```python
from build123d import *

# Parameters (mm, degrees)
SKETCH1_R               = 22.5
SKETCH1_R_2             = 20
BOSS_EXTRUDE1_DEPTH     = 30
BOSS_EXTRUDE2_DEPTH     = 4
CHAMFER1_SIZE           = 2
CHAMFER1_SIZE_2         = 1.79025908
CUT_EXTRUDE1_DEPTH      = 39.684622268
CUT_EXTRUDE1_DEPTH_BACK = 39.684622268
BOSS_EXTRUDE3_START     = -1.5
BOSS_EXTRUDE3_DEPTH     = 1.5
SKETCH6_R               = 13.5
SKETCH6_R_2             = 11.05
BOSS_EXTRUDE4_DEPTH     = 8
CHAMFER2_SIZE           = 1
CHAMFER3_SIZE           = 1
CHAMFER4_SIZE           = 2.5


with BuildPart() as part:
    # Sketch1 → Boss-Extrude1 (new body)
    with BuildSketch(Plane(origin=(0, 0, 0), x_dir=(1, 0, 0), z_dir=(0, 1, 0))):
        with Locations(Location((0, 0, 0), (0, 0, 270))):
            Circle(SKETCH1_R)
        with Locations(Location((0, 0, 0), (0, 0, 270))):
            Circle(SKETCH1_R_2, mode=Mode.SUBTRACT)
    extrude(amount=BOSS_EXTRUDE1_DEPTH)

    # Sketch2 → Boss-Extrude2 (add, symmetric)
    with BuildSketch(Plane(origin=(0, 18, 0), x_dir=(1, 0, 0), z_dir=(0, 1, 0))):
        with BuildLine():
            Line((-12.086630926, 15.934658856), (-4.330127019, 2.5))
            Line((-4.330127019, 2.5), (-19.843134833, 2.5))
            ThreePointArc((-19.843134833, 2.5), (-20, 0), (-19.843134833, -2.5))
            Line((-19.843134833, -2.5), (-4.330127019, -2.5))
            Line((-4.330127019, -2.5), (-12.086630926, -15.934658856))
            ThreePointArc((-12.086630926, -15.934658856), (-10, -17.320508076), (-7.756503907, -18.434658856))
            Line((-7.756503907, -18.434658856), (0, -5))
            Line((0, -5), (7.756503907, -18.434658856))
            ThreePointArc((7.756503907, -18.434658856), (10, -17.320508076), (12.086630926, -15.934658856))
            Line((12.086630926, -15.934658856), (4.330127019, -2.5))
            Line((4.330127019, -2.5), (19.843134833, -2.5))
            ThreePointArc((19.843134833, -2.5), (19.960745185, -1.252458251), (20, 0))
            ThreePointArc((20, 0), (19.960745185, 1.252458251), (19.843134833, 2.5))
            Line((19.843134833, 2.5), (4.330127019, 2.5))
            Line((4.330127019, 2.5), (12.086630926, 15.934658856))
            ThreePointArc((12.086630926, 15.934658856), (10, 17.320508076), (7.756503907, 18.434658856))
            Line((7.756503907, 18.434658856), (0, 5))
            Line((0, 5), (-7.756503907, 18.434658856))
            ThreePointArc((-7.756503907, 18.434658856), (-10, 17.320508076), (-12.086630926, 15.934658856))
        make_face()
    extrude(amount=BOSS_EXTRUDE2_DEPTH, both=True)

    # Chamfer1
    # the kernel refuses this chamfer: 2, 1.79025908 mm, written as the material it adds along each edge
    with BuildSketch(Plane(origin=(7.756503907, 22, 18.434658856), x_dir=(-0.9376749432180777, 0, 0.34751359809505994), z_dir=(0, -1, 0)), Plane(origin=(19.843134833, 22, 2.5), x_dir=(-0.16788186749818226, 0, 0.9858071203665161), z_dir=(0, -1, 0)), Plane(origin=(12.086630926, 22, -15.934658856), x_dir=(0.7697930757198956, 0, 0.6382935222714571), z_dir=(0, -1, 0)), Plane(origin=(-7.756503907, 22, -18.434658856), x_dir=(0.9376749432180783, 0, -0.34751359809505833), z_dir=(0, -1, 0)), Plane(origin=(-19.843134833, 22, -2.5), x_dir=(0.1678818674981782, 0, -0.9858071203665167), z_dir=(0, -1, 0)), Plane(origin=(-12.086630926, 22, 15.934658856), x_dir=(-0.7697930757198955, 0, -0.6382935222714572), z_dir=(0, -1, 0))) as chamfer1_piece_1:
        with BuildLine():
            Line((1.733569464, 0), (CHAMFER1_SIZE * 0.167881867498, CHAMFER1_SIZE * 0.985807120367))
            Line((CHAMFER1_SIZE * 0.167881867498, CHAMFER1_SIZE * 0.985807120367), (0, 0))
            ThreePointArc((0, 0), (0.889903139, -0.018778361), (1.733569464, 0))
        make_face()
    extrude(amount=8)
    with BuildSketch(Plane(origin=(12.086630926, 14, 15.934658856), x_dir=(0.7669529363679002, 0, -0.6417033531131466), z_dir=(0, 1, 0)), Plane(origin=(19.843134833, 14, -2.5), x_dir=(-0.17225493730569186, 0, -0.9850524029582447), z_dir=(0, 1, 0)), Plane(origin=(7.756503907, 14, -18.434658856), x_dir=(-0.9392078736735914, 0, -0.3433490498450975), z_dir=(0, 1, 0)), Plane(origin=(-12.086630926, 14, -15.934658856), x_dir=(-0.766952936367899, 0, 0.641703353113148), z_dir=(0, 1, 0)), Plane(origin=(-19.843134833, 14, 2.5), x_dir=(0.17225493730568892, 0, 0.9850524029582453), z_dir=(0, 1, 0)), Plane(origin=(-7.756503907, 14, 18.434658856), x_dir=(0.9392078736735913, 0, 0.3433490498450977), z_dir=(0, 1, 0))) as chamfer1_piece_2:
        with BuildLine():
            Line((1.910893878, 0), (CHAMFER1_SIZE_2 * 0.172254937261, CHAMFER1_SIZE_2 * 0.985052402702))
            Line((CHAMFER1_SIZE_2 * 0.172254937261, CHAMFER1_SIZE_2 * 0.985052402702), (0, 0))
            ThreePointArc((0, 0), (0.982338586, -0.022816928), (1.910893878, 0))
        make_face()
    extrude(amount=8)

    # Sketch4 → Cut-Extrude1 (cut, two sides: drawn at the far end of the back side and taken through both)
    with BuildSketch(Plane(origin=(0, 22, 0), x_dir=(1, 0, 0), z_dir=(0, 1, 0)).offset(-CUT_EXTRUDE1_DEPTH_BACK)):
        with BuildLine():
            Line((-1.09656677, 1.165135752), (-1.097544149, 0.833904576))
            Line((-1.097544149, 0.833904576), (-1.102446274, -0.827412964))
            Line((-1.102446274, -0.827412964), (-1.103423653, -1.15864414))
            ThreePointArc((-1.103423653, -1.15864414), (1.599993035, -0.004721172), (-1.09656677, 1.165135752))
        make_face()
    extrude(amount=CUT_EXTRUDE1_DEPTH + CUT_EXTRUDE1_DEPTH_BACK, mode=Mode.SUBTRACT)

    # Sketch5 → Boss-Extrude3 (add)
    with BuildSketch(Plane(origin=(0, 22, 0), x_dir=(1, 0, 0), z_dir=(0, 1, 0)).offset(BOSS_EXTRUDE3_START)):
        with BuildLine():
            Line((-1.09656677, 1.165135752), (-1.103423653, -1.15864414))
            ThreePointArc((-1.103423653, -1.15864414), (1.599993035, -0.004721172), (-1.09656677, 1.165135752))
        make_face()
    extrude(amount=BOSS_EXTRUDE3_DEPTH)

    # Sketch6 → Boss-Extrude4 (add)
    with BuildSketch(Plane(origin=(0, 22, 0), x_dir=(1, 0, 0), z_dir=(0, 1, 0))):
        with Locations(Location((0, 0, 0), (0, 0, 109.328070714))):
            Circle(SKETCH6_R)
        with Locations(Location((0, 0, 0), (0, 0, 73.076060846))):
            Circle(SKETCH6_R_2, mode=Mode.SUBTRACT)
    extrude(amount=BOSS_EXTRUDE4_DEPTH)

    # Chamfer2
    chamfer2_edges = [part.edges().sort_by_distance(p)[0] for p in [
        (0, 30, -22.5),
    ]]
    chamfer(chamfer2_edges, length=CHAMFER2_SIZE)

    # Chamfer3
    chamfer3_edges = [part.edges().sort_by_distance(p)[0] for p in [
        (-3.216676451, 30, 10.571447044),
    ]]
    chamfer(chamfer3_edges, length=CHAMFER3_SIZE)

    # Chamfer4
    # the kernel refuses this chamfer: 2.5 mm, written as the material it adds along each edge
    with BuildSketch(Plane(origin=(0, 22, 0), x_dir=(0.7884516512749685, 0, 0.6150967351577924), z_dir=(-0.6150967351577924, 0, 0.7884516512749685))) as chamfer4_piece_1_section:
        Polygon((13.5, CHAMFER4_SIZE), (13.5 + CHAMFER4_SIZE, 0), (13.5, 0), align=None)
    chamfer4_piece_1 = revolve(axis=Axis((0, 22, 0), (0, 1, 0)), revolution_arc=75.917899148, mode=Mode.PRIVATE)
    chamfer4_piece_1 = split(chamfer4_piece_1, bisect_by=Plane(origin=(0, 22, 2.5), z_dir=(0, 0, -1)), keep=Keep.TOP, mode=Mode.PRIVATE)
    chamfer4_piece_1 = split(chamfer4_piece_1, bisect_by=Plane(origin=(0, 22, -2.5), z_dir=(0, 0, 1)), keep=Keep.TOP, mode=Mode.PRIVATE)
    add(chamfer4_piece_1)
    with BuildSketch(Plane(origin=(0, 22, 0), x_dir=(0.9269152240690147, 0, -0.3752707920809829), z_dir=(0.3752707920809829, 0, 0.9269152240690147))) as chamfer4_piece_2_section:
        Polygon((13.5, CHAMFER4_SIZE), (13.5 + CHAMFER4_SIZE, 0), (13.5, 0), align=None)
    chamfer4_piece_2 = revolve(axis=Axis((0, 22, 0), (0, 1, 0)), revolution_arc=75.917899148, mode=Mode.PRIVATE)
    chamfer4_piece_2 = split(chamfer4_piece_2, bisect_by=Plane(origin=(2.165063509, 22, 1.25), z_dir=(-0.8660254037844385, 0, -0.5000000000000003)), keep=Keep.TOP, mode=Mode.PRIVATE)
    chamfer4_piece_2 = split(chamfer4_piece_2, bisect_by=Plane(origin=(-2.165063509, 22, -1.25), z_dir=(0.8660254037844383, 0, 0.5000000000000009)), keep=Keep.TOP, mode=Mode.PRIVATE)
    add(chamfer4_piece_2)
    with BuildSketch(Plane(origin=(0, 22, 0), x_dir=(0.138463572798161, 0, -0.9903675272382311), z_dir=(0.9903675272382311, 0, 0.138463572798161))) as chamfer4_piece_3_section:
        Polygon((13.5, CHAMFER4_SIZE), (13.5 + CHAMFER4_SIZE, 0), (13.5, 0), align=None)
    chamfer4_piece_3 = revolve(axis=Axis((0, 22, 0), (0, 1, 0)), revolution_arc=75.917899148, mode=Mode.PRIVATE)
    chamfer4_piece_3 = split(chamfer4_piece_3, bisect_by=Plane(origin=(-2.165063509, 22, 1.25), z_dir=(0.8660254037844393, 0, -0.49999999999999906)), keep=Keep.TOP, mode=Mode.PRIVATE)
    chamfer4_piece_3 = split(chamfer4_piece_3, bisect_by=Plane(origin=(2.165063509, 22, -1.25), z_dir=(-0.8660254037844392, 0, 0.49999999999999917)), keep=Keep.TOP, mode=Mode.PRIVATE)
    add(chamfer4_piece_3)
    with BuildSketch(Plane(origin=(0, 22, 0), x_dir=(-0.788451651274934, 0, -0.6150967351578366), z_dir=(0.6150967351578366, 0, -0.788451651274934))) as chamfer4_piece_4_section:
        Polygon((13.5, CHAMFER4_SIZE), (13.5 + CHAMFER4_SIZE, 0), (13.5, 0), align=None)
    chamfer4_piece_4 = revolve(axis=Axis((0, 22, 0), (0, 1, 0)), revolution_arc=75.917899148, mode=Mode.PRIVATE)
    chamfer4_piece_4 = split(chamfer4_piece_4, bisect_by=Plane(origin=(0, 22, -2.5), z_dir=(0, 0, 1)), keep=Keep.TOP, mode=Mode.PRIVATE)
    chamfer4_piece_4 = split(chamfer4_piece_4, bisect_by=Plane(origin=(0, 22, 2.5), z_dir=(0, 0, -1)), keep=Keep.TOP, mode=Mode.PRIVATE)
    add(chamfer4_piece_4)
    with BuildSketch(Plane(origin=(0, 22, 0), x_dir=(-0.9269152240690146, 0, 0.375270792080983), z_dir=(-0.375270792080983, 0, -0.9269152240690146))) as chamfer4_piece_5_section:
        Polygon((13.5, CHAMFER4_SIZE), (13.5 + CHAMFER4_SIZE, 0), (13.5, 0), align=None)
    chamfer4_piece_5 = revolve(axis=Axis((0, 22, 0), (0, 1, 0)), revolution_arc=75.917899148, mode=Mode.PRIVATE)
    chamfer4_piece_5 = split(chamfer4_piece_5, bisect_by=Plane(origin=(-2.165063509, 22, -1.25), z_dir=(0.8660254037844384, 0, 0.5000000000000006)), keep=Keep.TOP, mode=Mode.PRIVATE)
    chamfer4_piece_5 = split(chamfer4_piece_5, bisect_by=Plane(origin=(2.165063509, 22, 1.25), z_dir=(-0.8660254037844386, 0, -0.5000000000000003)), keep=Keep.TOP, mode=Mode.PRIVATE)
    add(chamfer4_piece_5)
    with BuildSketch(Plane(origin=(0, 22, 0), x_dir=(-0.13846357279405325, 0, 0.9903675272388054), z_dir=(-0.9903675272388054, 0, -0.13846357279405325))) as chamfer4_piece_6_section:
        Polygon((13.5, CHAMFER4_SIZE), (13.5 + CHAMFER4_SIZE, 0), (13.5, 0), align=None)
    chamfer4_piece_6 = revolve(axis=Axis((0, 22, 0), (0, 1, 0)), revolution_arc=75.917899148, mode=Mode.PRIVATE)
    chamfer4_piece_6 = split(chamfer4_piece_6, bisect_by=Plane(origin=(-2.165063509, 22, 1.25), z_dir=(0.8660254037844392, 0, -0.4999999999999992)), keep=Keep.TOP, mode=Mode.PRIVATE)
    chamfer4_piece_6 = split(chamfer4_piece_6, bisect_by=Plane(origin=(2.165063509, 22, -1.25), z_dir=(-0.866025403784439, 0, 0.4999999999999993)), keep=Keep.TOP, mode=Mode.PRIVATE)
    add(chamfer4_piece_6)


solid = part.part
```
Model file for the job. Use its own axes, mm. A direction names the side the tool comes from. Round coordinates to 2 decimals unless told otherwise and drop trailing zeros. Order: outer loops, then holes, each group sorted by start corner. A loop starts at its lowest first (then second) coordinate and runs counter-clockwise, first axis right, second up. Notation, with made-up numbers: (-26, 30.5) -> (26, 30.5) arc R27 ccw to (26, 64.5) -> close; hole circle Ø9 at (-32.5, 81.5). An arc over 180 degrees is marked (long way). Use one line per item in the form item = value.
Item 1: Tool access for faces 3 (the face through (11, 18, 2.5)), 4 (the face through (18.79, 17.94, -3.45)), 5 (the face through (-19, 22, 0)): list every direction of +Z, -Z, +X, -X, +Y, -Y with a clear straight run to the whole face (end or side of a thin tool).
Returned:
face_3 = -Y
face_4 = +Y, -Y
face_5 = +Y
Item 2: Drill centre lines: line 1 (X direction, y = 27.5, z = 0); line 2 (Z direction, x = -11, y = 19.5); line 3 (X direction, y = 15.5, z = 0). Where is each one in solid material? Low to high.
Returned:
line_1 = -22.5 to -20, -13.5 to -11.05, 11.05 to 13.5, 20 to 22.5
line_2 = -19.63 to -14.05, -2.5 to 2.5, 14.05 to 19.63
line_3 = -22.5 to -1.1, 1.6 to 22.5
Item 3: Cut at B-B, the plane y = 10.25. Write the cut outline in (x, z), and give its area (3 significant figures).
Returned:
outline = circle Ø45 at (0, 0); hole circle Ø40 at (0, 0)
area = 334 mm^2
Item 4: Flat gauge pins, fed straight in: pin 1 Ø8 at (x, y) = (8, 4.5) entering from -Z; pin 2 Ø7.5 at (x, z) = (-10.5, 16.5) entering from +Y; pin 3 Ø2 at (x, z) = (17.5, -1) entering from +Y; pin 4 Ø1.7 at (x, z) = (-10.5, -8) entering from -Y. Where does each tip first touch, or does it go through?
Returned:
pin_1 = -22.14
pin_2 = 30
pin_3 = 22
pin_4 = 22
Item 5: Cut at C-C, the plane x = -2.5. Give the number of separate pieces and of enclosed holes in the cut face, and give its area (3 significant figures).
Returned:
separate_pieces = 5
enclosed_holes = 0
area = 338 mm^2
Item 6: Pull direction X, two halves, no side cores. Call faces 1 (the face through (-6, 30, 11)), 2 (the face through (11, 22, -6)): released by +X, released by -X, zero draft, split by the parting line, or undercut.
Returned:
face_1 = zero draft
face_2 = undercut
